```python
from build123d import *

# Parameters (mm, degrees)
F0_W     = 25.4
F0_H     = 12.7
F1_DEPTH = 25.4
F3_DEPTH = 25.4


with BuildPart() as f1:
    # F0 (on Top) → F1 (new body)
    with BuildSketch(Plane.XY):
        with Locations((12.7, 6.35)):
            Rectangle(F0_W, F0_H)
    extrude(amount=F1_DEPTH)

    # F2 (on face) → F3 (join)
    with BuildSketch(Plane(origin=(0, 12.7, 0), x_dir=(-1, 0, 0), z_dir=(0, 1, 0))):
        with BuildLine():
            Line((-12.7, 12.7), (-6.9540247637, 12.7))
            ThreePointArc((-6.9540247637, 12.7), (-16.7630180541, 16.7630180541), (-12.7, 6.9540247637))
            Line((-12.7, 6.9540247637), (-12.7, 12.7))
        make_face()
    extrude(amount=F3_DEPTH)


solid = f1.part
```
Check sheet for the modelled part. Datum: model origin and axes. Units: mm. A direction names the side the tool comes from. Round coordinates to 2 decimals unless told otherwise and drop trailing zeros. Write each loop counter-clockwise with the first axis right and the second up, starting at its lowest first coordinate (ties: lowest second). Pieces come first, ordered by that corner, then holes. Notation, with made-up numbers: (61.5, -18) -> (116.5, -18) arc R27 ccw to (116.5, 17) -> close; hole circle Ø1 at (84.5, -39.5). An arc over 180 degrees is marked (long way). One line per question, with ' | ' between items. Start each with the question number.
1. Sectioned sample at A-A, the plane x = 14. Record the cut outline in (y, z).
2. Depth check by flat-ended pin: pin 1 (1 mm diameter, centred on x = 14, y = 23.5, fed in from -Z); pin 2 (4.5 mm diameter, centred on x = 8.5, y = 29, fed in from -Z); pin 3 (8 mm diameter, centred on x = 7.5, z = 2.5, fed in from +Y); pin 4 (1 mm diameter, centred on y = 30, z = 6, fed in from -X). Enter the tip coordinate at first touch or a pass-through.
3. Sectioned sample at C-C, the plane y = 35. Record the cut outline in (x, z).
4. Set-up check for faces 1 (the face through (16.63, 25.22, 16.89)), 2 (the face through (13, 38.1, 13)), 3 (the face through (10, 25, 12.7)): record each of +Z, -Z, +X, -X, +Y, -Y from which the full face is reachable in a straight line by a thin tool's end or side.
5. Scan lines: line 1 along Y through (x, z) = (5.75, 5.75); line 2 along X through (y, z) = (26, 13); line 3 along Z through (x, y) = (9.25, 23). Record each from-to range of solid material in increasing order. Write a range as from..to.
6. Sectioned sample at B-B, the plane z = 11. Record the cut outline in (x, y), then the cut area to 3 significant figures.
7. Sectioned sample at D-D, the plane x = 19.5. Record the cut outline in (y, z).
Taken from the geometry:
1) outline: (0, 0) -> (12.7, 0) -> (12.7, 7.1) -> (38.1, 7.1) -> (38.1, 18.3) -> (12.7, 18.3) -> (12.7, 25.4) -> (0, 25.4) -> close
2) pin 1: stops at z = 7.01 | pin 2: stops at z = 12.7 | pin 3: stops at y = 12.7 | pin 4: passes through
3) outline: (6.95, 12.7) -> (12.7, 12.7) -> (12.7, 6.95) arc R5.75 ccw (long way) to start
4) face 1: +Y | face 2: +Z, -Z, +X, -X, +Y | face 3: -Z, -X, +Y
5) line 1: y = 0..12.7 | line 2: x = 6.96..18.44 | line 3: z = 12.7..17.29
6) outline: (0, 0) -> (25.4, 0) -> (25.4, 12.7) -> (18.19, 12.7) -> (18.19, 38.1) -> (12.7, 38.1) -> (12.7, 12.7) -> (0, 12.7) -> close | area: 462 mm^2
7) outline: (0, 0) -> (12.7, 0) -> (12.7, 25.4) -> (0, 25.4) -> close
